Geometry: final body of the model. Coordinates: model frame, mm. A direction names the side the tool comes from. Give positions to 0.01 mm unless a question says otherwise; leave off trailing zeros. Loops run counter-clockwise (first coordinate to the right, second up) from the corner with the lowest first, then second, coordinate; pieces in that order, holes last. Notation, with made-up numbers: (36, -18) -> (73, -18) arc R26 cw to (73, 18) -> close; hole circle Ø5 at (-5.75, 17.5). An arc over 180 degrees is marked (long way). Answer in a Markdown table with one row per item. Add a question column.
from build123d import *

# Parameters (mm, degrees)
BOX3525_W        = 1300
BOX3525_H        = 550
BOX3525_DEPTH    = 500
ARRAY280_Z_COUNT = 4
ARRAY280_Z_PITCH = 550
BOX3524_W        = 1400
BOX3524_H        = 600
BOX3524_DEPTH    = 2200


with BuildPart() as array280:
    # Box3525 → Box3525 (new body)
    with BuildSketch(Plane(origin=(8750, -1950, 0), x_dir=(1, 0, 0), z_dir=(0, 0, 1))):
        with Locations((650, 275)):
            Rectangle(BOX3525_W, BOX3525_H)
    extrude(amount=BOX3525_DEPTH)

    # Array280 Z: Array280 ×4


with BuildPart() as array280_1:
    add(array280.part)
    with Locations(*[(0, 0, i * ARRAY280_Z_PITCH) for i in range(1, ARRAY280_Z_COUNT)]):
        add(array280.part)


with BuildPart() as cut002:
    # Box3524 → Box3524 (new body)
    with BuildSketch(Plane(origin=(8700, -2000, 0), x_dir=(1, 0, 0), z_dir=(0, 0, 1))):
        with Locations((700, 300)):
            Rectangle(BOX3524_W, BOX3524_H)
    extrude(amount=BOX3524_DEPTH)

    # Cut002: cut Array280
    add(array280_1.part, mode=Mode.SUBTRACT)


solid = cut002.part
(1) Pin query (flat end, axial travel): pin 1 Ø3 at (x, z) = (9027, 1883) entering from +Y. Return the tip coordinate at first contact, or that it passes through.
(2) Cut plane B-B on z = 1553.5. Return the cut outline in (x, y).
(3) Cut plane A-A on y = -1927.5. Return the cut outline in (x, z), then the cut area to 3 significant figures.
(4) Cut plane C-C on x = 9180. Return the cut outline in (y, z).
(5) Reachability of faces 4 (the flat face through (8750, -1679, 246)), 5 (the flat face through (9391, -1671, 1600)), 6 (the flat face through (9397, -1965, 0)) from +Z, -Z, +X, -X, +Y, -Y: full face, straight path, thin tool, end or side. Return the list, or none.
(6) Draft query along Z for faces 1 (the flat face through (10050, -1679, 246)), 2 (the flat face through (10050, -1679, 796)), 3 (the flat face through (9391, -1671, 500)). Return one class per face: +Z half, -Z half, draft (parallel to the pull), parting line (faces both ways), or undercut.
(7) Material intervals for line 1 along Z through (x, y) = (9880.5, -1889); line 2 along X through (y, z) = (-1645, 488); line 3 along Y through (x, z) = (9244, 584), sorted ascending. Write a range as from..to.
Answer list:
| question | item | result |
|---|---|---|
| 1 | pin 1 | stops at y = -1950 |
| 2 | outline | (8700, -2000) -> (10100, -2000) -> (10100, -1400) -> (10050, -1400) -> (10050, -1950) -> (8750, -1950) -> (8750, -1400) -> (8700, -1400) -> close |
| 3 | outline | (8700, 0) -> (8750, 0) -> (8750, 500) -> (10050, 500) -> (10050, 0) -> (10100, 0) -> (10100, 2200) -> (8700, 2200) -> close; hole (8750, 550) -> (10050, 550) -> (10050, 1050) -> (8750, 1050) -> close; hole (8750, 1100) -> (10050, 1100) -> (10050, 1600) -> (8750, 1600) -> close; hole (8750, 1650) -> (10050, 1650) -> (10050, 2150) -> (8750, 2150) -> close |
| 3 | area | 480,000 mm² |
| 4 | outline | (-2000, 0) -> (-1950, 0) -> (-1950, 500) -> (-1400, 500) -> (-1400, 550) -> (-1950, 550) -> (-1950, 1050) -> (-1400, 1050) -> (-1400, 1100) -> (-1950, 1100) -> (-1950, 1600) -> (-1400, 1600) -> (-1400, 1650) -> (-1950, 1650) -> (-1950, 2150) -> (-1400, 2150) -> (-1400, 2200) -> (-2000, 2200) -> close |
| 5 | face 4 | -Z, +Y |
| 5 | face 5 | +Y |
| 5 | face 6 | -Z, +X, -X, +Y, -Y |
| 6 | face 1 | draft |
| 6 | face 2 | undercut |
| 6 | face 3 | -Z half |
| 7 | line 1 | z = 500..550, 1050..1100, 1600..1650, 2150..2200 |
| 7 | line 2 | x = 8700..8750, 10050..10100 |
| 7 | line 3 | y = -2000..-1950 |
